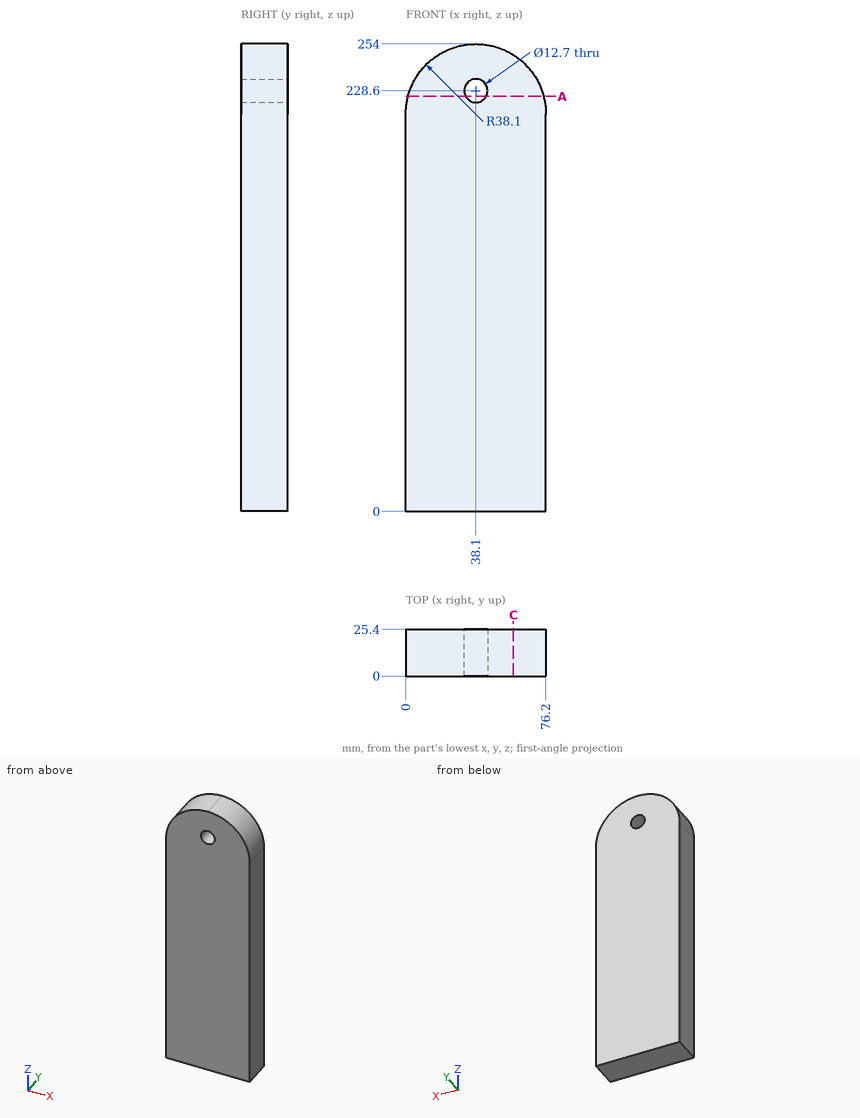
Input: dimensioned drawing with shaded views. Units: mm. Origin: part minimum x, y, z. Round coordinates to 2 decimals unless told otherwise and drop trailing zeros. Order: outer loops, then holes, each group sorted by start corner. A loop starts at its lowest first (then second) coordinate and runs counter-clockwise, first axis right, second up. Notation, with made-up numbers: M 31.25,-10.5 L 90.25,-10.5 A3 ccw 90.25,-6.5 Z; hole C -9,3.5 d5. An arc over 180 degrees is marked long. Use one line per item in the form item = value. Start each with the question number.
Q1. Cut plane C-C (x = 58.5). Return loops of the section in (y, z), and give its area (3 significant figures).
Q2. Pin query (flat end, axial travel): pin 1 Ø12 at (x, y) = (24.5, 18) entering from +Z; pin 2 Ø1 at (x, y) = (56.5, 11) entering from +Z. Return the tip coordinate at first contact, or that it passes through.
Q3. Cut plane A-A (z = 225.5). Return loops of the section in (x, y), and give its area (3 significant figures).
Q4. Material intervals for line 1 (Z direction, x = 42.5, y = 12.5); line 2 (Z direction, x = 39, y = 20); line 3 (Z direction, x = 60, y = 2.25), sorted ascending. Write a range as [from, to].
Geometry results:
q1.outline = M 0,0 L 25.4,0 L 25.4,248.08 L 0,248.08 Z
q1.area = 6,300 mm^2
q2.pin_1 = 253.23
q2.pin_2 = 249.53
q3.outline = M 1.23,0 L 32.56,0 L 32.56,25.4 L 1.23,25.4 Z; M 43.64,0 L 74.97,0 L 74.97,25.4 L 43.64,25.4 Z
q3.area = 1,590 mm^2
q4.line_1 = [0, 224.02], [233.18, 253.75]
q4.line_2 = [0, 222.31], [234.89, 253.99]
q4.line_3 = [0, 247.08]
